from build123d import *

# Parameters (mm, degrees)
SKETCH5_R           = 5
BOSS_EXTRUDE2_DEPTH = 2


with BuildPart() as part:
    # Sketch1 → Revolve1 (revolve)
    with BuildSketch(Plane(origin=(0, 0, 0), x_dir=(1, 0, 0), z_dir=(0, 1, 0))):
        with BuildLine():
            Line((12.781543507, 13.383116119), (-2.50303312, 13.383116119))
            ThreePointArc((-2.50303312, 13.383116119), (-2.501361875, 13.293526957), (-2.506133274, 13.204049335))
            Line((-2.506133274, 13.204049335), (-2.506133274, 9.63773694))
            Line((-2.506133274, 9.63773694), (0, 9.63773694))
            Line((0, 9.63773694), (0, 3.705))
            Line((0, 3.705), (0, 0))
            Line((0, 0), (4.789576981, 0))
            Line((4.789576981, 0), (4.808638309, 3.705))
            ThreePointArc((4.808638309, 3.705), (5.009621244, 3.664180843), (5.185678757, 3.558994837))
            ThreePointArc((5.185678757, 3.558994837), (7.965698705, 8.014106646), (12.465543511, 10.721121396))
            ThreePointArc((12.465543511, 10.721121396), (12.633558311, 10.915283437), (12.780786925, 11.125644095))
            Line((12.780786925, 11.125644095), (12.781543507, 13.383116119))
        make_face()
    revolve(axis=Axis((0, 0, 0), (1, 0, 0)))

    # Sketch2 → Revolved-Cut2 (revolve, cut)
    with BuildSketch(Plane.ZY.offset(-12.773866726)):
        Polygon((13.385193973, 0), (-13.385193973, 0), (-16.077753665, 0), (-16.077753665, 11.5), (15.518432284, 11.5), (15.518432284, 0), align=None)
    revolve(axis=Axis((12.773866726, 0, -16.077753665), (0, 0, 1)), mode=Mode.SUBTRACT)

    # Sketch5 → Boss-Extrude2 (add)
    with BuildSketch(Plane.ZY):
        Circle(SKETCH5_R)
    extrude(amount=BOSS_EXTRUDE2_DEPTH)


solid = part.part
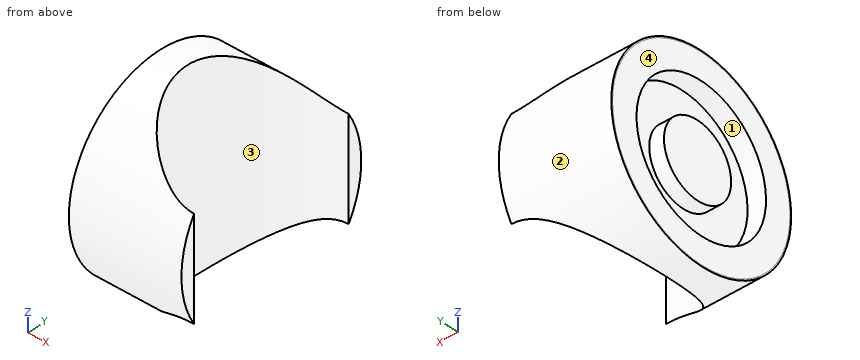
Could you check a few things on this model? Use its own coordinates, in mm. Face numbers are marked on the shaded views. Coordinates: 2 decimals unless noted, no trailing zeros. Order: outer loops, then holes, each group sorted by start corner. A loop starts at its lowest first (then second) coordinate and runs counter-clockwise, first axis right, second up. Notation, with made-up numbers: (37, 17) - (64, 17) arc R31 ccw to (64, 55) - close; hole circle Ø2 at (6.25, 71.5). An arc over 180 degrees is marked (long way). Answer in a Markdown table with one row per item. Add a question column.
(1) I need wall thicknesses on L1, parallel to Y at x = -1.8, z = 0; L2, parallel to Y at x = 3.75, z = -7.25; L3, parallel to Y at x = 10.5, z = 3.75. Which ranges of each line are inside material? Lowest first, please.
(2) If we section it at A-A, the plane x = -0.5: Please give me the cut outline in (y, z), then the cut area to 3 significant figures.
(3) Will these pins go through, and if not, where does the flat tip stop? pin 1 (4 mm diameter, centred on x = 7.5, z = 5.5, fed in from +Y); pin 2 (4 mm diameter, centred on x = 5, y = 4, fed in from -Z); pin 3 (8 mm diameter, centred on x = 2.5, z = -1.5, fed in from -Y); pin 4 (2 mm diameter, centred on x = 7.5, z = -1.5, fed in from +Y).
(4) If we mould it in two halves opening along Y, with no side actions, what happens to the marked faces 1, 2, 3 and 4? For each: released by +Y, released by -Y, zero draft, split by the parting line, or undercut.
(5) If we section it at B-B, the plane z = 0: Please give me the cut outline in (x, y).
(6) If we section it at C-C, the plane y = 0: Please give me the cut outline in (x, z), then the cut area to 3 significant figures.
(7) If we section it at D-D, the plane x = 5: Please give me the cut outline in (y, z).
Results are:
| question | item | result |
|---|---|---|
| 1 | L1 | y = -13.38 to -9.64, -5 to 5, 9.64 to 13.38 |
| 1 | L2 | y = -11.25 to -7.13, 7.13 to 11.25 |
| 1 | L3 | y = -12.85 to -11.27, 11.27 to 12.85 |
| 2 | outline | circle Ø26.77 at (0, 0); circle Ø10 at (0, 0); hole circle Ø19.28 at (0, 0) |
| 2 | area | 349 mm2 |
| 3 | pin 1 | stops at y = 12.92 |
| 3 | pin 2 | passes through |
| 3 | pin 3 | stops at y = -13.38 |
| 3 | pin 4 | stops at y = 13.37 |
| 4 | face 1 | undercut |
| 4 | face 2 | split by the parting line |
| 4 | face 3 | undercut |
| 4 | face 4 | zero draft |
| 5 | outline | (-2.51, -13.2) arc R1.25 cw to (-2.5, -13.38) - (12.78, -13.38) - (12.78, -11.5) arc R11.5 cw to (12.78, 11.5) - (12.78, 13.38) - (-2.5, 13.38) arc R1.25 cw to (-2.51, 13.2) - (-2.51, 9.64) - (0, 9.64) - (0, 5) - (-2, 5) - (-2, -5) - (0, -5) - (0, -9.64) - (-2.51, -9.64) - close |
| 6 | outline | (-2.51, -13.2) arc R1.25 cw to (-2.5, -13.38) - (1.27, -13.38) - (1.27, 13.38) - (-2.5, 13.38) arc R1.25 cw to (-2.51, 13.2) - (-2.51, 9.64) - (0, 9.64) - (0, 5) - (-2, 5) - (-2, -5) - (0, -5) - (0, -9.64) - (-2.51, -9.64) - close |
| 6 | area | 72.9 mm2 |
| 7 | outline | (-8.47, -10.36) - (-8.47, 10.36) arc R13.38 ccw to start; (8.47, -10.36) arc R13.38 ccw to (8.47, 10.36) - close |
